Verification items for this drawing (mm, ordinates from the low corner). A direction names the side the tool comes from. Give positions to 0.01 mm unless a question says otherwise; leave off trailing zeros. Loops run counter-clockwise (first coordinate to the right, second up) from the corner with the lowest first, then second, coordinate; pieces in that order, holes last. Notation, with made-up numbers: (-12, -4) -> (22, -4) arc R22 cw to (22, 27) -> close; hole circle Ø9 at (-21, -2.5). An arc over 180 degrees is marked (long way). Use one line per item in the form item = value. Start each with the question number.
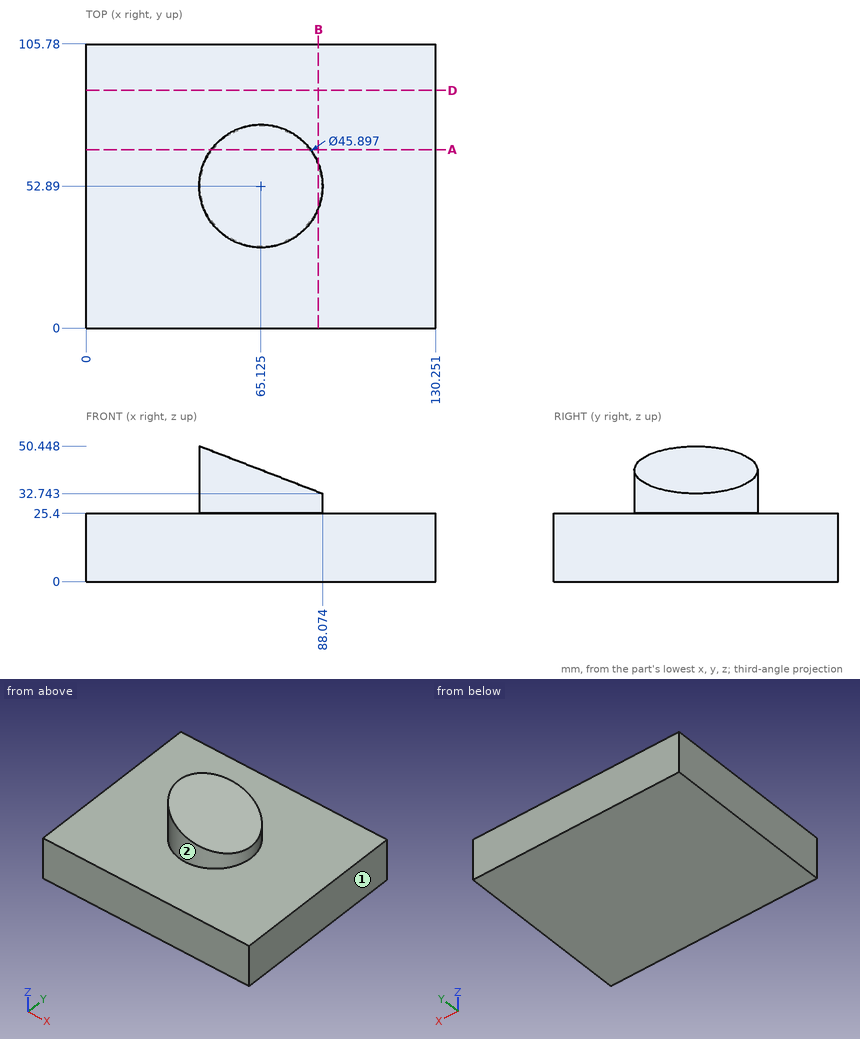
Item 1: Sectioned sample at A-A, the plane y = 66.5. Enter the section's corners in (x, z), and give its area (3 significant figures).
Item 2: Sectioned sample at D-D, the plane y = 88.5. Enter the section's corners in (x, z), and give its area (3 significant figures).
Item 3: Sectioned sample at B-B, the plane x = 86.5. Enter the section's corners in (y, z), and give its area (3 significant figures).
Item 4: Gauge pin test, flat ends, axial feed: pin 1 Ø1.5 at (y, z) = (74.5, 35) entering from +X; pin 2 Ø4 at (y, z) = (70, 28.5) entering from -X (1 decimal); pin 3 Ø1.5 at (x, z) = (45.5, 34) entering from +Y; pin 4 Ø4 at (y, z) = (89.5, 24.5) entering from -X. Record the tip position at first contact, or that the pin passes through.
Item 5: Tool access check on the marked faces 1 and 2. Record the directions out of +Z, -Z, +X, -X, +Y, -Y that give a thin tool (end or side, any length) a straight path to the whole face; none if there is none.
Item 6: Material ranges on line 1 (Z direction, x = 61, y = 11.5); line 2 (Y direction, x = 63, z = 41); line 3 (Z direction, x = 58.5, y = 71), recorded low to high.
Outcome:
q1.outline = (0, 0) -> (130.25, 0) -> (130.25, 25.4) -> (83.6, 25.4) -> (83.6, 34.47) -> (46.65, 48.72) -> (46.65, 25.4) -> (0, 25.4) -> close
q1.area = 3,910 mm^2
q2.outline = (0, 0) -> (130.25, 0) -> (130.25, 25.4) -> (0, 25.4) -> close
q2.area = 3,310 mm^2
q3.outline = (0, 0) -> (105.78, 0) -> (105.78, 25.4) -> (61.24, 25.4) -> (61.24, 33.35) -> (44.54, 33.35) -> (44.54, 25.4) -> (0, 25.4) -> close
q3.area = 2,820 mm^2
q4.pin_1 = 74.69
q4.pin_2 = 47.9
q4.pin_3 = 65.94
q4.pin_4 = 0
q5.face_1 = +Z, -Z, +X, +Y, -Y
q5.face_2 = +Z
q6.line_1 = 0 to 25.4
q6.line_2 = 30.04 to 75.74
q6.line_3 = 0 to 44.15
